Here's how the part is built. I have some questions about the finished solid (model axes, mm). Round coordinates to 2 decimals unless told otherwise and drop trailing zeros. Loops run counter-clockwise (first coordinate to the right, second up) from the corner with the lowest first, then second, coordinate; pieces in that order, holes last. Notation, with made-up numbers: (74, 42.25) - (92, 42.25) arc R22 cw to (92, 79.25) - close; hole circle Ø8 at (61.25, -33). An arc over 180 degrees is marked (long way). Answer as a JSON object with one key per item and string values. Group by question number.
1) Will these pins go through, and if not, where does the flat tip stop? P1, Ø6, axis at x = 29, z = 15.5, coming from the -Y side; P2, Ø8, axis at y = 11.5, z = 4.5, coming from the -X side; P3, Ø8, axis at x = 33, z = 16.5, coming from the +Y side.
2) I want a section at D-D, the plane x = 23.5. Please give me the cut outline in (y, z).
3) If I drill on line 1 along Z through (x, y) = (14.5, 8); line 2 along Z through (x, y) = (33.5, 13); line 3 along Y through (x, z) = (46, 17.75), over which ranges is the centre line in solid material (lowest first)? Write a range as [from, to].
4) I want a section at C-C, the plane z = 15. Please give me the cut outline in (x, y), then the cut area to 3 significant figures.
5) I want a section at B-B, the plane y = 11. Please give me the cut outline in (x, z), then the cut area to 3 significant figures.
6) I want a section at A-A, the plane y = 23. Please give me the cut outline in (x, z), then the cut area to 3 significant figures.
from build123d import *

# Parameters (mm, degrees)
F1_R     = 1.6
F2_DEPTH = 2.5
F3_W     = 7
F3_H     = 18.5
F4_DEPTH = 2.5
F5_R     = 1.6
F6_DEPTH = 2.5


with BuildPart() as f2:
    # F1 (on offset) → F2 (new body)
    with BuildSketch(Plane.XY.offset(16)):
        with BuildLine():
            ThreePointArc((48.0560038294, 18.8446410406), (49.5170345112, 20.1361157487), (50.0602513075, 22.0089299644))
            ThreePointArc((50.0602513075, 22.0089299644), (48.4330655233, 24.9657131681), (45.0644987857, 25.1732188883))
            ThreePointArc((45.0644987857, 25.1732188883), (43.3959623837, 20.5131774426), (48.0560038294, 18.8446410406))
        make_face()
        with Locations((46.5602513075, 22.0089299644)):
            Circle(F1_R, mode=Mode.SUBTRACT)
        with BuildLine():
            ThreePointArc((48.0560038294, 18.8446410406), (43.3959623837, 20.5131774426), (45.0644987857, 25.1732188883))
            Line((45.0644987857, 25.1732188883), (21.7843731319, 14.168753906))
            Line((21.7843731319, 14.168753906), (24.7758781756, 7.8401760584))
            Line((24.7758781756, 7.8401760584), (48.0560038294, 18.8446410406))
        make_face()
    extrude(amount=F2_DEPTH)

    # F3 (on face) → F4 (join)
    with BuildSketch(Plane(origin=(23.2801256538, 11.0044649822, 0), x_dir=(0.4273578634, -0.9040825497, 0), z_dir=(-0.9040825497, -0.4273578634, 0))):
        with Locations((0, 9.25)):
            Rectangle(F3_W, F3_H)
    extrude(amount=F4_DEPTH)

    # F5 (on Top) → F6 (join)
    with BuildSketch(Plane.XY):
        with BuildLine():
            ThreePointArc((-3.0246602264, -5.3010782407), (-1.5636295447, -4.0096035327), (-1.0204127483, -2.1367893169))
            ThreePointArc((-1.0204127483, -2.1367893169), (-2.6475985325, 0.8199938867), (-6.0161652702, 1.0274996069))
            ThreePointArc((-6.0161652702, 1.0274996069), (-7.6847016721, -3.6325418388), (-3.0246602264, -5.3010782407))
        make_face()
        with Locations((-4.5204127483, -2.1367893169)):
            Circle(F5_R, mode=Mode.SUBTRACT)
        with BuildLine():
            ThreePointArc((-6.0161652702, 1.0274996069), (-2.6475985325, 0.8199938867), (-1.0204127483, -2.1367893169))
            ThreePointArc((-1.0204127483, -2.1367893169), (-1.5636295447, -4.0096035327), (-3.0246602264, -5.3010782407))
            Line((-3.0246602264, -5.3010782407), (22.5156718015, 6.7717813999))
            Line((22.5156718015, 6.7717813999), (19.5241667578, 13.1003592476))
            Line((19.5241667578, 13.1003592476), (-6.0161652702, 1.0274996069))
        make_face()
    extrude(amount=F6_DEPTH)


solid = f2.part
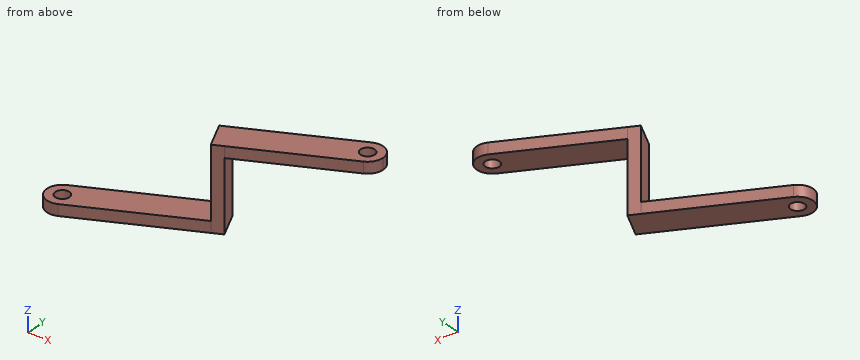
Outcome:
{
 "1": {"P1": "y = 8.44", "P2": "x = 8.81", "P3": "y = 21.36"},
 "2": {"outline": "(7.24, 0) - (10.54, 0) - (10.54, 16) - (14.98, 16) - (14.98, 18.5) - (7.24, 18.5) - close"},
 "3": {"line 1": "[0, 2.5]", "line 2": "[16, 18.5]", "line 3": "[17.87, 20.51], [23.51, 25.46]"},
 "4": {"outline": "(19.52, 13.1) - (22.52, 6.77) - (24.78, 7.84) - (21.78, 14.17) - close", "area": "17.5 mm^2"},
 "5": {"outline": "(15.08, 0) - (23.28, 0) - (23.28, 16) - (31.46, 16) - (31.46, 18.5) - (20.52, 18.5) - (20.52, 2.5) - (15.08, 2.5) - close", "area": "85.2 mm^2"},
 "6": {"outline": "(40.47, 16) - (45.3, 16) - (45.3, 18.5) - (40.47, 18.5) - close; (47.82, 16) - (49.92, 16) - (49.92, 18.5) - (47.82, 18.5) - close", "area": "17.3 mm^2"}
}
